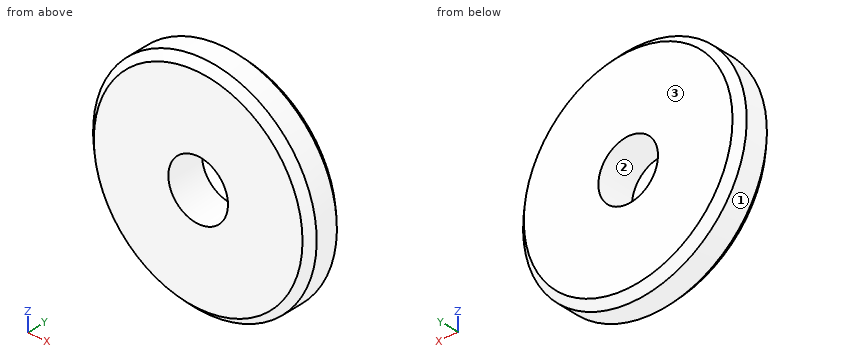
```python
from build123d import *

# Parameters (mm, degrees)
SKETCH_1_R          = 15
EXTRUDE_1_DEPTH     = 5
CHAMFER_1_SIZE      = 1
SKETCH_2_R          = 4
CUT_EXTRUDE_1_DEPTH = 22.794494718


with BuildPart() as part:
    # 草图1 → 凸台-拉伸1 (new body)
    with BuildSketch(Plane(origin=(0, 0, 0), x_dir=(1, 0, 0), z_dir=(0, 1, 0))):
        with Locations(Location((0, 0, 0), (0, 0, 270))):
            Circle(SKETCH_1_R)
    extrude(amount=EXTRUDE_1_DEPTH)

    # 倒角1
    chamfer_1_edges = [part.edges().sort_by_distance(p)[0] for p in [
        (0, 0, -15),
        (0, 5, -15),
    ]]
    chamfer(chamfer_1_edges, length=CHAMFER_1_SIZE)

    # 草图2 → 切除-拉伸1 (cut, through all)
    with BuildSketch(Plane.XZ):
        with Locations(Location((0, 0, 0), (0, 0, 270))):
            Circle(SKETCH_2_R)
    extrude(amount=-CUT_EXTRUDE_1_DEPTH, mode=Mode.SUBTRACT)


solid = part.part
```
Work out the finished part from the listing and answer in its coordinate system (mm). Face numbers are marked on the shaded views. Coordinates: 2 decimals unless noted, no trailing zeros. Loops run counter-clockwise (first coordinate to the right, second up) from the corner with the lowest first, then second, coordinate; pieces in that order, holes last. Notation, with made-up numbers: (70, 56) -> (129, 56) arc R28 ccw to (129, 95) -> close; hole circle Ø6 at (4.25, 65). An arc over 180 degrees is marked (long way). Answer as CSV lines item,"result".
Q1. The part is cut by section A-A on z = 0. Write down the section's boundary in (x, y).
Findings:
outline,"(-15, 1) -> (-14, 0) -> (-4, 0) -> (-4, 5) -> (-14, 5) -> (-15, 4) -> close; (4, 0) -> (14, 0) -> (15, 1) -> (15, 4) -> (14, 5) -> (4, 5) -> close"
Q2. Find the intervals of material crossed by probe 1 along X at (y, z) = (1.1, 0); probe 2 along X at (y, z) = (0.8, 3.5); probe 3 along Y at (x, z) = (-7, 12.25), in increasing order.
Findings:
probe 1,"x = -15 to -4, 4 to 15"
probe 2,"x = -14.38 to -1.94, 1.94 to 14.38"
probe 3,"y = 0.11 to 4.89"
Q3. For a pull along Z with two mould halves and no side action, classify the marked faces 1, 2 and 3 as +Z half, -Z half, draft (parallel to the pull), parting line (faces both ways), or undercut.
Findings:
face 1,"parting line"
face 2,"undercut"
face 3,"draft"
Q4. The part is cut by section B-B on x = 0. Write down the section's boundary in (y, z).
Findings:
outline,"(0, -14) -> (1, -15) -> (4, -15) -> (5, -14) -> (5, -4) -> (0, -4) -> close; (0, 4) -> (5, 4) -> (5, 14) -> (4, 15) -> (1, 15) -> (0, 14) -> close"
Q5. Each of these flat-tipped pins is pushed along its axis until it touches: pin 1 (1.5 mm diameter, centred on y = 4, z = 10, fed in from +X); pin 2 (2 mm diameter, centred on y = 3, z = 5, fed in from +X). Where does it stop, or does it pass through?
Findings:
pin 1,"stops at x = 11.81"
pin 2,"stops at x = 14.46"
Q6. The part is cut by section C-C on y = 3.25. Write down the section's boundary in (x, z), and give its area (3 significant figures).
Findings:
outline,"circle Ø30 at (0, 0); hole circle Ø8 at (0, 0)"
area,"657 mm²"
